Design review of the part shown in the three views and the two pictorial views. Dimensions are in mm from the part's minimum x, y and z. Coordinates: 2 decimals unless noted, no trailing zeros. Loops run counter-clockwise (first coordinate to the right, second up) from the corner with the lowest first, then second, coordinate; pieces in that order, holes last. Notation, with made-up numbers: (-22.5, 79) -> (-13.5, 79) arc R16 ccw to (-13.5, 103) -> close; hole circle Ø10 at (36, 41). An arc over 180 degrees is marked (long way). Answer in a Markdown table with one row per item.
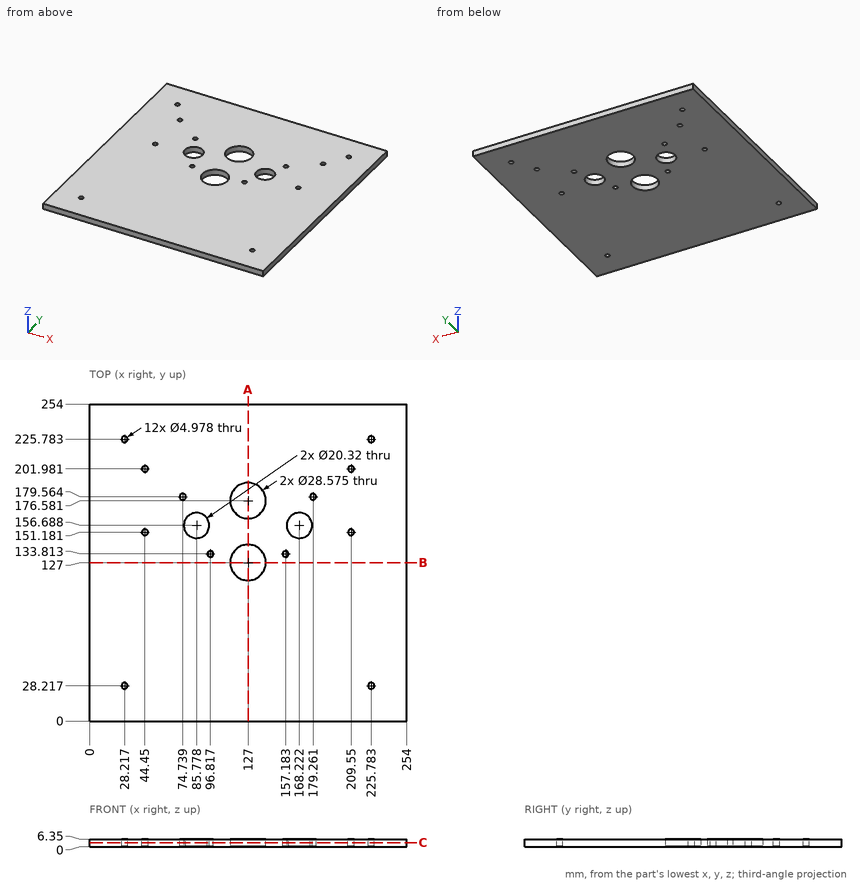
Item 1: Insertion check: pin 1 (2 mm diameter, centred on x = 126.5, y = 154, fed in from -Z); pin 2 (3 mm diameter, centred on x = 74.74, y = 179.56, fed in from -Z). Each pin has a flat end and moves straight along its axis. Give the tip position at first contact, or say it passes through.
Worked answers:
| item | result |
|---|---|
| pin 1 | z = 0 |
| pin 2 | through |
Item 2: Take a section at B-B, the plane y = 127. State the section outline as (x, z) points.
Worked answers:
| item | result |
|---|---|
| outline | (0, 0) -> (112.71, 0) -> (112.71, 6.35) -> (0, 6.35) -> close; (141.29, 0) -> (254, 0) -> (254, 6.35) -> (141.29, 6.35) -> close |
Item 3: Take a section at A-A, the plane x = 127. State the section outline as (y, z) points.
Worked answers:
| item | result |
|---|---|
| outline | (0, 0) -> (112.71, 0) -> (112.71, 6.35) -> (0, 6.35) -> close; (141.29, 0) -> (162.29, 0) -> (162.29, 6.35) -> (141.29, 6.35) -> close; (190.87, 0) -> (254, 0) -> (254, 6.35) -> (190.87, 6.35) -> close |
Item 4: For L1, parallel to X at y = 155.5, z = 4; L2, parallel to X at y = 132.5, z = 5.75 (1 decimal); L3, parallel to Y at x = 27, z = 3 (1 decimal), list the stretches that pass through material, from the lowest coordinate up.
Worked answers:
| item | result |
|---|---|
| L1 | 0 to 75.69, 95.87 to 158.13, 178.31 to 254 |
| L2 | 0 to 94.7, 98.9 to 113.8, 140.2 to 155.1, 159.3 to 254 |
| L3 | 0 to 26, 30.4 to 223.6, 228 to 254 |
Item 5: Take a section at C-C, the plane z = 3.5. Count the separate pieces of the cut face and the enclosed holes in it, and give its area (4 significant figures).
Worked answers:
| item | result |
|---|---|
| separate pieces | 1 |
| enclosed holes | 16 |
| area | 62,350 mm² |
